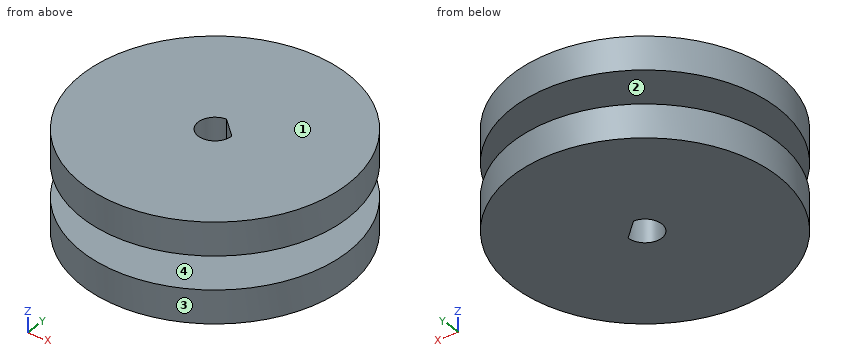
```python
from build123d import *

# Parameters (mm, degrees)
F0_R     = 20
F1_DEPTH = 5
F2_R     = 5
F3_DEPTH = 5
F4_R     = 20
F5_DEPTH = 5
F7_DEPTH = 25


with BuildPart() as f1:
    # F0 (on Top) → F1 (new body)
    with BuildSketch(Plane.XY):
        Circle(F0_R)
    extrude(amount=F1_DEPTH)

    # F2 (on face) → F3 (join)
    with BuildSketch(Plane.XY.offset(5)):
        Circle(F2_R)
    extrude(amount=F3_DEPTH)

    # F4 (on face) → F5 (join)
    with BuildSketch(Plane.XY.offset(10)):
        Circle(F4_R)
    extrude(amount=F5_DEPTH)

    # F6 (on face) → F7 (cut)
    with BuildSketch(Plane.XY.offset(15)):
        with BuildLine():
            ThreePointArc((-0.1480392157, 2.5456991948), (-1.75, -1.8547236991), (2.55, 0))
            Line((2.55, 0), (-0.1480392157, 2.5456991948))
        make_face()
    extrude(amount=-F7_DEPTH, mode=Mode.SUBTRACT)


solid = f1.part
```
Can you work these out from the model? Positions are in its coordinate system, mm. Face numbers are marked on the shaded views. Give positions to 0.01 mm unless a question says otherwise; leave off trailing zeros. Order: outer loops, then holes, each group sorted by start corner. A loop starts at its lowest first (then second) coordinate and runs counter-clockwise, first axis right, second up. Notation, with made-up numbers: (61, 69) - (65, 69) arc R21 cw to (65, 91) - close; hole circle Ø4 at (18.25, -38). An arc over 180 degrees is marked (long way). Use a Markdown table: item, result. Add a question column.
Q1. I'm going to push flat-ended pins straight in: pin 1 (1.5 mm diameter, centred on y = 8, z = 5.5, fed in from -X); pin 2 (8 mm diameter, centred on x = 8, z = 6.5, fed in from -Y); pin 3 (1.5 mm diameter, centred on y = -11, z = 12, fed in from +X). Where does each tip first touch, or does it pass through?
Q2. Please list where these lines run through material, in increasing order: line 1 along Z through (x, y) = (1, 5); line 2 along Y through (x, z) = (0, 3.5); line 3 along Y through (x, z) = (0.5, 1.5).
Q3. If we section it at B-B on y = 13: Write out the boundary of the cut face in (x, z).
Q4. If we section it at A-A on x = 12: Write out the boundary of the cut face in (y, z).
Q5. If we section it at D-D on x = -4: Write out the boundary of the cut face in (y, z), plus the area to 3 significant figures.
Q6. If we section it at C-C on z = 11.25: Write out the boundary of the cut face in (x, y), plus the area to 3 significant figures.
Q7. If we mould it in two halves opening along Z, with no side actions, what happens to the marked faces 1, 2, 3 and 4? For each: released by +Z, released by -Z, zero draft, split by the parting line, or undercut.
Answers follow:
| question | item | result |
|---|---|---|
| 1 | pin 1 | stops at x = -18.56 |
| 1 | pin 2 | stops at y = -19.53 |
| 1 | pin 3 | stops at x = 17.17 |
| 2 | line 1 | z = 0 to 5, 10 to 15 |
| 2 | line 2 | y = -20 to -2.55, 2.41 to 20 |
| 2 | line 3 | y = -19.99 to -2.5, 1.93 to 19.99 |
| 3 | outline | (-15.2, 0) - (15.2, 0) - (15.2, 5) - (-15.2, 5) - close; (-15.2, 10) - (15.2, 10) - (15.2, 15) - (-15.2, 15) - close |
| 4 | outline | (-16, 0) - (16, 0) - (16, 5) - (-16, 5) - close; (-16, 10) - (16, 10) - (16, 15) - (-16, 15) - close |
| 5 | outline | (-19.6, 0) - (19.6, 0) - (19.6, 5) - (3, 5) - (3, 10) - (19.6, 10) - (19.6, 15) - (-19.6, 15) - (-19.6, 10) - (-3, 10) - (-3, 5) - (-19.6, 5) - close |
| 5 | area | 422 mm^2 |
| 6 | outline | circle Ø40 at (0, 0); hole (-0.15, 2.55) arc R2.55 ccw (long way) to (2.55, 0) - close |
| 6 | area | 1,240 mm^2 |
| 7 | face 1 | released by +Z |
| 7 | face 2 | undercut |
| 7 | face 3 | zero draft |
| 7 | face 4 | undercut |
